Here's how the part is built. I have some questions about the finished solid (model axes, mm). A direction names the side the tool comes from. Give positions to 0.01 mm unless a question says otherwise; leave off trailing zeros. Order: outer loops, then holes, each group sorted by start corner. A loop starts at its lowest first (then second) coordinate and runs counter-clockwise, first axis right, second up. Notation, with made-up numbers: (-26, -2) - (0, -2) arc R17 ccw to (0, 3) - close; hole circle Ø10 at (21.5, 74.5). An arc over 180 degrees is marked (long way). One line per question, with ' | ' between items.
from build123d import *

# Parameters (mm, degrees)
F1_DEPTH = 63.5
F2_R     = 3.048
F3_DEPTH = 2.9972
F5_R     = 3.175
F4_R     = 3.175
F6_DEPTH = 25.4
F7_SIZE  = 1.27
F8_R     = 2.54
F9_R     = 1.27


with BuildPart() as f1:
    # F0 (on Top) → F1 (new body)
    with BuildSketch(Plane.XY):
        Polygon((4.5752139781, 0), (-9.0290260219, 0), (-9.0290260219, 13.59535), (-24.9040260219, 13.59535), (-24.9040260219, 10.42035), (-12.2040260219, 10.42035), (-12.2040260219, -5.92963), (7.7502139781, -5.92963), (7.7502139781, 10.42035), (20.4502139781, 10.42035), (20.4502139781, 13.59535), (4.5752139781, 13.59535), align=None)
    extrude(amount=F1_DEPTH)

    # F2 (on face) → F3 (cut)
    with BuildSketch(Plane(origin=(0, 0, 0), x_dir=(-1, 0, 0), z_dir=(0, 1, 0))):
        with Locations((2.2269060219, 31.75)):
            Circle(F2_R)
    extrude(amount=-F3_DEPTH, mode=Mode.SUBTRACT)

    # F5 (on face) + F4 (on face) → F6 (cut)
    with BuildSketch(Plane(origin=(0, 13.59535, 0), x_dir=(-1, 0, 0), z_dir=(0, 1, 0))):
        with Locations((-13.5922139781, 49.0982)):
            Circle(F5_R)
        with Locations((-13.5922139781, 14.4018)):
            Circle(F5_R)
    with BuildSketch(Plane(origin=(0, 13.59535, 0), x_dir=(-1, 0, 0), z_dir=(0, 1, 0))):
        with Locations((18.0460260219, 49.0982)):
            Circle(F4_R)
        with Locations((18.0460260219, 14.4018)):
            Circle(F4_R)
    extrude(amount=-F6_DEPTH, mode=Mode.SUBTRACT)

    # F7
    f7_edges = [f1.edges().sort_by_distance(p)[0] for p in [
        (-14.871026, 10.42035, 49.0982),
        (-14.871026, 10.42035, 14.4018),
        (16.767214, 10.42035, 49.0982),
        (16.767214, 10.42035, 14.4018),
    ]]
    chamfer(f7_edges, length=F7_SIZE)

    # F8
    f8_edges = [f1.edges().sort_by_distance(p)[0] for p in [
        (7.750214, -5.92963, 31.75),
        (-12.204026, -5.92963, 31.75),
    ]]
    fillet(f8_edges, radius=F8_R)

    # F9
    f9_edges = [f1.edges().sort_by_distance(p)[0] for p in [
        (-9.029026, 6.797675, 63.5),
        (4.575214, 6.797675, 63.5),
        (-2.226906, 0, 63.5),
    ]]
    fillet(f9_edges, radius=F9_R)


solid = f1.part
1) Please list where these lines run through material, in increasing order: L1, parallel to X at y = 9, z = 20; L2, parallel to X at y = 12.5, z = 33; L3, parallel to Y at x = 17, z = 55.
Model answer:
L1: x = -12.2 to -9.03, 4.58 to 7.75 | L2: x = -24.9 to -9.03, 4.58 to 20.45 | L3: y = 10.42 to 13.6
2) I'm going to push flat-ended pins straight in: P1, Ø10, axis at y = 4, z = 37.5, coming from the +X side; P2, Ø4, axis at x = -16.5, z = 19.5, coming from the -Y side; P3, Ø5, axis at x = -2.5, z = 33, coming from the +Y side. Where does each tip first touch, or does it pass through?
Model answer:
P1: stops at x = 7.75 | P2: stops at y = 10.42 | P3: stops at y = 0
3) I want a section at D-D (x = -17). State how many separate pieces and enclosed holes the cut face has, plus the area to 3 significant figures.
Model answer:
separate pieces: 3 | enclosed holes: 0 | area: 160 mm2
4) I want a section at B-B (x = -6). List the corners of the cut face in (y, z) for me.
Model answer:
outline: (-5.93, 0) - (0, 0) - (0, 62.23) arc R1.27 ccw to (-1.27, 63.5) - (-5.93, 63.5) - close
5) On a 3-axis mill with a long thin cutter (end or side, diameter ignored), from which of +Z, -Z, +X, -X, +Y, -Y can I reach the whole of each face in a straight line? I mean faces 4 (the face through (-12.204, 4, 31)), 5 (the face through (4.575, 7, 31)), 6 (the face through (-2.34, -0.362, 63.118)), 7 (the face through (14, 10.42, 31)). Say none if no direction works.
Model answer:
face 4: +Z, -Z, -X, -Y | face 5: +Z, -Z, +Y | face 6: +Z, +Y | face 7: +Z, -Z, +X, -Y
6) Thinking about a two-plate mould opening in Z: for faces 1 (the face through (1, 0, 31)), 2 (the face through (-9.391, 6.267, 63.118)), 3 (the face through (14.28, 12.66, 46)), which applies, +Z half, -Z half, draft (parallel to the pull), parting line (faces both ways), or undercut?
Model answer:
face 1: draft | face 2: +Z half | face 3: undercut
7) I want a section at C-C (z = 31.75). List the corners of the cut face in (x, y) for me.
Model answer:
outline: (-24.9, 10.42) - (-12.2, 10.42) - (-12.2, -3.39) arc R2.54 ccw to (-9.66, -5.93) - (5.21, -5.93) arc R2.54 ccw to (7.75, -3.39) - (7.75, 10.42) - (20.45, 10.42) - (20.45, 13.6) - (4.58, 13.6) - (4.58, 0) - (0.82, 0) - (0.82, -3) - (-5.27, -3) - (-5.27, 0) - (-9.03, 0) - (-9.03, 13.6) - (-24.9, 13.6) - close
8) I want a section at A-A (y = 3). List the corners of the cut face in (x, z) for me.
Model answer:
outline: (-12.2, 0) - (-9.03, 0) - (-9.03, 62.23) arc R1.27 ccw to (-10.3, 63.5) - (-12.2, 63.5) - close; (4.58, 0) - (7.75, 0) - (7.75, 63.5) - (5.85, 63.5) arc R1.27 ccw to (4.58, 62.23) - close
